```python
from build123d import *

# Parameters (mm, degrees)
SKETCH_1_W          = 110
SKETCH_1_H          = 78
SKETCH_1_R          = 1.6
EXTRUDE_1_DEPTH     = 3
FILLET_1_R          = 3
SKETCH_2_R          = 2
CUT_EXTRUDE_1_DEPTH = 10
SKETCH_3_R          = 2.5
CUT_EXTRUDE_2_DEPTH = 10


with BuildPart() as part:
    # 草图1 → 凸台-拉伸1 (new body)
    with BuildSketch(Plane(origin=(0, 0, 0), x_dir=(1, 0, 0), z_dir=(0, 1, 0))):
        Rectangle(SKETCH_1_W, SKETCH_1_H)
        with Locations(Location((-37, 36, 0), (0, 0, 270))):
            Circle(SKETCH_1_R, mode=Mode.SUBTRACT)
        with Locations(Location((37, 36, 0), (0, 0, 270))):
            Circle(SKETCH_1_R, mode=Mode.SUBTRACT)
        with Locations(Location((37, -36, 0), (0, 0, 270))):
            Circle(SKETCH_1_R, mode=Mode.SUBTRACT)
        with Locations(Location((-37, -36, 0), (0, 0, 270))):
            Circle(SKETCH_1_R, mode=Mode.SUBTRACT)
    extrude(amount=EXTRUDE_1_DEPTH)

    # 圆角1
    fillet_1_edges = [part.edges().sort_by_distance(p)[0] for p in [
        (-55, 1.5, -39),
        (55, 1.5, -39),
        (55, 1.5, 39),
        (-55, 1.5, 39),
    ]]
    fillet(fillet_1_edges, radius=FILLET_1_R)

    # 草图2 → 切除-拉伸1 (cut)
    with BuildSketch(Plane(origin=(0, 3, 0), x_dir=(1, 0, 0), z_dir=(0, 1, 0))):
        with Locations(Location((-14, 5, 0), (0, 0, 270))):
            Circle(SKETCH_2_R)
        with Locations(Location((35, 5, 0), (0, 0, 270))):
            Circle(SKETCH_2_R)
        with Locations(Location((35, -5, 0), (0, 0, 270))):
            Circle(SKETCH_2_R)
        with Locations(Location((-14, -5, 0), (0, 0, 270))):
            Circle(SKETCH_2_R)
    extrude(amount=-CUT_EXTRUDE_1_DEPTH, mode=Mode.SUBTRACT)

    # 草图3 → 切除-拉伸2 (cut)
    with BuildSketch(Plane.XZ):
        with Locations(Location((-26.110622524, 0, 0), (0, 0, 270))):
            Circle(SKETCH_3_R)
        with Locations(Location((13.889377476, 0, 0), (0, 0, 270))):
            Circle(SKETCH_3_R)
    extrude(amount=-CUT_EXTRUDE_2_DEPTH, mode=Mode.SUBTRACT)


solid = part.part
```
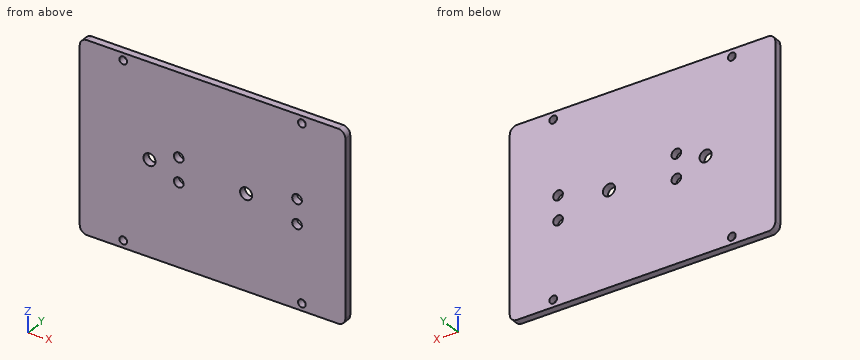
Input: part model. Units: mm. Frame: model coordinates. Coordinates: 2 decimals unless noted, no trailing zeros. Write each loop counter-clockwise with the first axis right and the second up, starting at its lowest first coordinate (ties: lowest second). Pieces come first, ordered by that corner, then holes. Notation, with made-up numbers: (9.25, 48.25) -> (32.25, 48.25) arc R26 ccw to (32.25, 76.25) -> close; hole circle Ø5 at (86, -18.5). An arc over 180 degrees is marked (long way). Answer as a JSON object with one key per item and string values.
1. Section B-B on z = 5. Return the cut outline in (x, y), then the cut area to 3 significant figures.
Result set:
{"outline": "(-55, 0) -> (-16, 0) -> (-16, 3) -> (-55, 3) -> close; (-12, 0) -> (33, 0) -> (33, 3) -> (-12, 3) -> close; (37, 0) -> (55, 0) -> (55, 3) -> (37, 3) -> close", "area": "306 mm2"}
2. Material intervals for line 1 (X direction, y = 2.4, z = -36); line 2 (X direction, y = 1.9, z = 0); line 3 (Z direction, x = -25, y = 2.6), sorted ascending. Write a range as from..to.
Result set:
{"line 1": "x = -55..-38.6, -35.4..35.4, 38.6..55", "line 2": "x = -55..-28.61, -23.61..11.39, 16.39..55", "line 3": "z = -39..-2.24, 2.24..39"}
3. Section A-A on x = -37. Return the cut outline in (y, z).
Result set:
{"outline": "(0, -39) -> (3, -39) -> (3, -37.6) -> (0, -37.6) -> close; (0, -34.4) -> (3, -34.4) -> (3, 34.4) -> (0, 34.4) -> close; (0, 37.6) -> (3, 37.6) -> (3, 39) -> (0, 39) -> close"}
4. First-contact query: P1, Ø5, axis at x = 35, z = 5, coming from the +Y side. Flat tip, straight axial feed; report the tip coordinate or a pass-through.
Result set:
{"P1": "stops at y = 3"}
5. Section C-C on y = 0.65. Count the separate pieces of the cut face and the enclosed holes in it, then the cut area to 3 significant figures.
Result set:
{"separate pieces": "1", "enclosed holes": "10", "area": "8,450 mm2"}
